Could you check a few things on this model? Use its own coordinates, in mm. A direction names the side the tool comes from. Give positions to 0.01 mm unless a question says otherwise; leave off trailing zeros. Write each loop counter-clockwise with the first axis right and the second up, starting at its lowest first coordinate (ties: lowest second). Pieces come first, ordered by that corner, then holes. Notation, with made-up numbers: (6, 4) - (23, 4) arc R28 ccw to (23, 34) - close; hole circle Ø6 at (16.5, 6). An arc over 180 degrees is marked (long way). Answer in a Markdown table with one row per item.
from build123d import *

# Parameters (mm, degrees)
SKETCH_1_R      = 11
EXTRUDE_1_DEPTH = 10


with BuildPart() as part:
    # Эскиз1 → Вытянуть1 (new body)
    with BuildSketch(Plane(origin=(0, 0, 0), x_dir=(1, 0, 0), z_dir=(0, 1, 0))):
        with BuildLine():
            Line((-34.176272466, 48.057375978), (105.823727534, 48.057375978))
            Line((105.823727534, 48.057375978), (105.823727534, 2.562145774))
            Line((105.823727534, 2.562145774), (79.601322316, 2.562145774))
            ThreePointArc((79.601322316, 2.562145774), (76.06578841, 1.09767968), (74.601322316, -2.437854226))
            Line((74.601322316, -2.437854226), (74.601322316, -31.447393818))
            ThreePointArc((74.601322316, -31.447393818), (76.06578841, -34.982927724), (79.601322316, -36.447393818))
            Line((79.601322316, -36.447393818), (105.823727534, -36.447393818))
            Line((105.823727534, -36.447393818), (105.823727534, -81.942624022))
            Line((105.823727534, -81.942624022), (-34.176272466, -81.942624022))
            Line((-34.176272466, -81.942624022), (-34.176272466, -36.447393818))
            Line((-34.176272466, -36.447393818), (-7.953867248, -36.447393818))
            ThreePointArc((-7.953867248, -36.447393818), (-4.418333342, -34.982927724), (-2.953867248, -31.447393818))
            Line((-2.953867248, -31.447393818), (-2.953867248, -2.437854226))
            ThreePointArc((-2.953867248, -2.437854226), (-4.418333342, 1.09767968), (-7.953867248, 2.562145774))
            Line((-7.953867248, 2.562145774), (-34.176272466, 2.562145774))
            Line((-34.176272466, 2.562145774), (-34.176272466, 48.057375978))
        make_face()
        with Locations(Location((35.823727534, -16.942624022, 0), (0, 0, 270))):
            Circle(SKETCH_1_R, mode=Mode.SUBTRACT)
    extrude(amount=EXTRUDE_1_DEPTH)


solid = part.part
1) Imagine slicing it at C-C (y = 3). List the corners of the cut face in (x, z) for me.
Check values:
| item | result |
|---|---|
| outline | (-34.18, -48.06) - (105.82, -48.06) - (105.82, -2.56) - (79.6, -2.56) arc R5 cw to (74.6, 2.44) - (74.6, 31.45) arc R5 cw to (79.6, 36.45) - (105.82, 36.45) - (105.82, 81.94) - (-34.18, 81.94) - (-34.18, 36.45) - (-7.95, 36.45) arc R5 cw to (-2.95, 31.45) - (-2.95, 2.44) arc R5 cw to (-7.95, -2.56) - (-34.18, -2.56) - close; hole circle Ø22 at (35.82, 16.94) |
2) We'd pull the mould along Z, two halves only. Please class faces 1 (the face through (74.601, 5, 17)), 2 (the face through (37, 5, 81.943)), 3 (the face through (-34.176, 5, -25)), 4 (the face through (-2.954, 5, 17)): +Z half, -Z half, draft (parallel to the pull), parting line (faces both ways), or undercut.
Check values:
| item | result |
|---|---|
| face 1 | undercut |
| face 2 | +Z half |
| face 3 | draft |
| face 4 | undercut |
3) Imagine slicing it at A-A (x = -17). List the corners of the cut face in (y, z) for me.
Check values:
| item | result |
|---|---|
| outline | (0, -48.06) - (10, -48.06) - (10, -2.56) - (0, -2.56) - close; (0, 36.45) - (10, 36.45) - (10, 81.94) - (0, 81.94) - close |
4) Will this pin go through, and if not, where does the flat tip stop? P1, Ø5, axis at y = 6.5, z = 27, coming from the +X side.
Check values:
| item | result |
|---|---|
| P1 | stops at x = 74.6 |
5) If I drill on line 1 (Z direction, x = -8.5, y = 8.25); line 2 (Z direction, x = 76, y = 8.25); line 3 (X direction, y = 5.5, z = 13), over which ranges is the centre line in solid material (lowest first)?
Check values:
| item | result |
|---|---|
| line 1 | z = -48.06 to -2.56, 36.45 to 81.94 |
| line 2 | z = -48.06 to -1.03, 34.92 to 81.94 |
| line 3 | x = -2.95 to 25.55, 46.09 to 74.6 |
6) Imagine slicing it at B-B (z = 17.5). List the corners of the cut face in (x, y) for me, then the cut area to 3 significant figures.
Check values:
| item | result |
|---|---|
| outline | (-2.95, 0) - (24.84, 0) - (24.84, 10) - (-2.95, 10) - close; (46.81, 0) - (74.6, 0) - (74.6, 10) - (46.81, 10) - close |
| area | 556 mm2 |
7) On a 3-axis mill with a long thin cutter (end or side, diameter ignored), from which of +Z, -Z, +X, -X, +Y, -Y can I reach the whole of each face in a straight line? I mean faces 5 (the face through (105.824, 5, -26)), 6 (the face through (76.027, 4.93, 34.944)), 7 (the face through (-21, 5, -2.562)). Say none if no direction works.
Check values:
| item | result |
|---|---|
| face 5 | +Z, -Z, +X, +Y, -Y |
| face 6 | +X, +Y, -Y |
| face 7 | -X, +Y, -Y |
